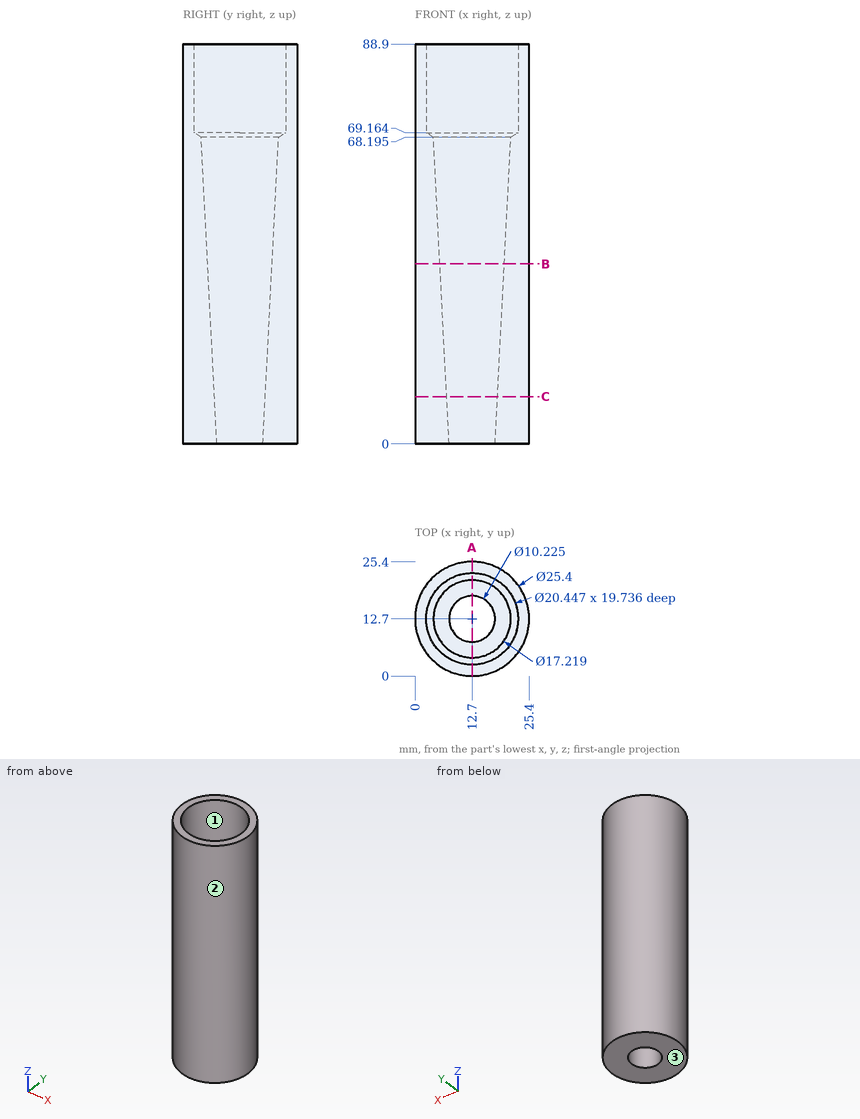
Geometry: see drawing. Coordinates: mm, zero at the bounding-box minimum. Coordinates: 2 decimals unless noted, no trailing zeros. Loops run counter-clockwise (first coordinate to the right, second up) from the corner with the lowest first, then second, coordinate; pieces in that order, holes last. Notation, with made-up numbers: (-31.5, 67) - (-17.5, 67) arc R31 cw to (-17.5, 101) - close; hole circle Ø7 at (39, 59). An arc over 180 degrees is marked (long way). Return JSON: item names as keys, results as strings.
Q1. Section A-A, the plane x = 12.7. Return loops of the section in (y, z) (1 decimal).
Results:
{"outline": "(0, 0) - (7.6, 0) - (4.1, 68.2) - (2.5, 69.2) - (2.5, 88.9) - (0, 88.9) - close; (17.8, 0) - (25.4, 0) - (25.4, 88.9) - (22.9, 88.9) - (22.9, 69.2) - (21.3, 68.2) - close"}
Q2. Section C-C, the plane z = 10.5. Return loops of the section in (x, y), plus the area to 3 significant figures.
Results:
{"outline": "circle Ø25.4 at (12.7, 12.7); hole circle Ø11.3 at (12.7, 12.7)", "area": "406 mm2"}
Q3. Section B-B, the plane z = 40. Return loops of the section in (x, y).
Results:
{"outline": "circle Ø25.4 at (12.7, 12.7); hole circle Ø14.33 at (12.7, 12.7)"}
Q4. Contact query for flat-ended pins moving along their axis: P1, Ø5, axis at x = 22, z = 15.5, coming from the -Y side (1 decimal); P2, Ø1.5, axis at x = 14, y = 20.5, coming from the +Z side; P3, Ø1, axis at x = 5.5, z = 15, coming from the +Y side. Output: stop coordinate, or through.
Results:
{"P1": "y = 2", "P2": "z = 68.22", "P3": "y = 23.49"}
Q5. Material intervals for line 1 along Y through (x, z) = (12.7, 78.5); line 2 along X through (y, z) = (7.25, 34); line 3 along X through (y, z) = (18.75, 45) (1 decimal), sorted ascending.
Results:
{"line 1": "0 to 2.48, 22.92 to 25.4", "line 2": "1.23 to 8.54, 16.86 to 24.17", "line 3": "1.5 to 8.4, 17 to 23.9"}
Q6. Mould query, pull axis X, two halves, no side actions, for the marked faces 1, 2 and 3. Classes: released by +X, released by -X, zero draft, split by the parting line, or undercut.
Results:
{"face 1": "undercut", "face 2": "split by the parting line", "face 3": "zero draft"}
